```python
from build123d import *

# Parameters (mm, degrees)
SKETCH1_W           = 22.5
SKETCH1_H           = 30
SKETCH1_W_2         = 7.5
SKETCH1_H_2         = 7.5
BOSS_EXTRUDE1_DEPTH = 5
CUT_EXTRUDE1_DEPTH  = 51.698249477


with BuildPart() as part:
    # Sketch1 → Boss-Extrude1 (new body)
    with BuildSketch(Plane(origin=(0, 0, 0), x_dir=(1, 0, 0), z_dir=(0, 1, 0))):
        Polygon((-11.25, 7.5), (-11.25, 15), (-33.75, 15), (-33.75, 0), (-26.25, 0), (-26.25, 7.5), align=None)
        Rectangle(SKETCH1_W, SKETCH1_H)
        with Locations((0, 18.75)):
            Rectangle(SKETCH1_W_2, SKETCH1_H_2)
        Polygon((18.75, 15), (11.25, 15), (11.25, 7.5), (26.25, 7.5), (26.25, 27.813163598), (33.75, 27.813163598), (33.75, 35.313163598), (18.75, 35.313163598), align=None)
        Polygon((11.25, -15), (3.75, -15), (3.75, -22.5), (26.25, -22.5), (26.25, -30), (33.75, -30), (33.75, -15), align=None)
        Polygon((-3.75, -15), (-11.25, -15), (-11.25, -22.5), (-26.25, -22.5), (-26.25, -37.5), (-18.75, -37.5), (-18.75, -30), (-3.75, -30), align=None)
    extrude(amount=BOSS_EXTRUDE1_DEPTH)

    # Sketch2 → Cut-Extrude1 (cut, through all)
    with BuildSketch(Plane(origin=(0, 5, 0), x_dir=(1, 0, 0), z_dir=(0, 1, 0))):
        Polygon((0, 7.5), (-5.25, 0), (0, -7.5), (5.25, 0), align=None)
    extrude(amount=-CUT_EXTRUDE1_DEPTH, mode=Mode.SUBTRACT)


solid = part.part
```
For this review, take the finished solid that the model builds, in its own axes (mm). A direction names the side the tool comes from. Coordinates: 2 decimals unless noted, no trailing zeros. Loops run counter-clockwise (first coordinate to the right, second up) from the corner with the lowest first, then second, coordinate; pieces in that order, holes last.
1. Insertion check: P1, Ø1.5, axis at y = 1.5, z = -2, coming from the +X side; P2, Ø2.5, axis at x = -30.5, y = 3, coming from the +Z side; P3, Ø1.5, axis at x = -1.5, y = 3.5, coming from the +Z side. Each pin has a flat end and moves straight along its axis. Give the tip position at first contact, or say it passes through.
2. Add section B-B, the plane x = 23. Give the boundary of the cut face in (y, z), then the cut area to 3 significant figures.
3. Mouldability with a two-part tool opening along Z and no side actions: class faces 4 (the flat face through (-26.25, 2, -4)), 5 (the flat face through (0, 2, 15)), 6 (the flat face through (33.75, 2, 23)) as +Z half, -Z half, draft (parallel to the pull), parting line (faces both ways), or undercut.
4. Add section A-A, the plane z = 18. Give the boundary of the cut face in (x, y), then the cut area to 4 significant figures.
5. Add section D-D, the plane z = -30. Give the boundary of the cut face in (x, y).
6. For faces 1 (the flat face through (11, 2, -15)), 2 (the flat face through (-26.25, 2, 30)), 3 (the flat face through (26.25, 2, -18)), list the 3-axis set-ups (+Z, -Z, +X, -X, +Y, -Y) from which the entire face can be reached by the end or side of a thin tool; tool diameter is ignored.
7. For line 1 (X direction, y = 4.5, z = -17); line 2 (Z direction, x = 11.5, y = 2); line 3 (Z direction, x = -11.5, y = 1.1), list the stretches that pass through material, from the lowest coordinate up.
Result:
1. P1: stops at x = 11.25
1. P2: stops at z = 0
1. P3: stops at z = 15
2. outline: (0, -35.31) - (5, -35.31) - (5, -7.5) - (0, -7.5) - close; (0, 15) - (5, 15) - (5, 22.5) - (0, 22.5) - close
2. area: 177 mm2
3. face 4: undercut
3. face 5: +Z half
3. face 6: draft
4. outline: (-11.25, 0) - (-3.75, 0) - (-3.75, 5) - (-11.25, 5) - close; (3.75, 0) - (33.75, 0) - (33.75, 5) - (3.75, 5) - close
4. area: 187.5 mm2
5. outline: (18.75, 0) - (33.75, 0) - (33.75, 5) - (18.75, 5) - close
6. face 1: -Z, +Y, -Y
6. face 2: +Z, -X, +Y, -Y
6. face 3: +X, +Y, -Y
7. line 1: x = -3.75 to 3.75, 18.75 to 26.25
7. line 2: z = -15 to -7.5, 15 to 22.5
7. line 3: z = -15 to -7.5, 22.5 to 30
